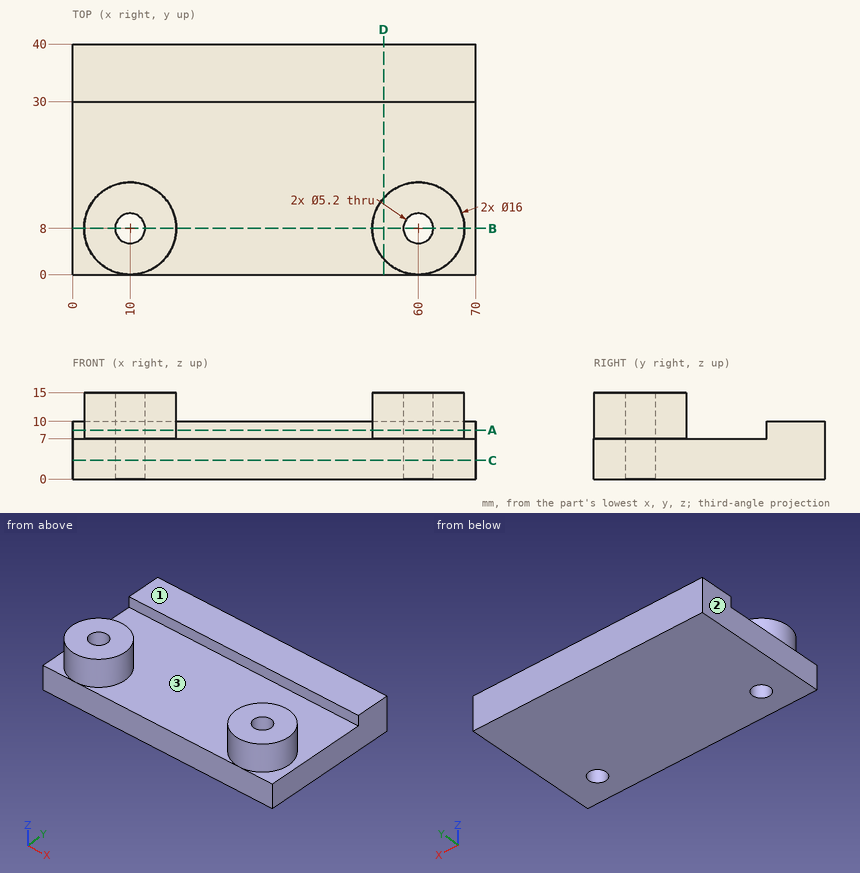
Could you check a few things on this drawing? It's one solid part, dimensions in mm from its lowest x, y, z. A direction names the side the tool comes from. Round coordinates to 2 decimals unless told otherwise and drop trailing zeros. Order: outer loops, then holes, each group sorted by start corner. A loop starts at its lowest first (then second) coordinate and runs counter-clockwise, first axis right, second up. Notation, with made-up numbers: M 4.5,-24.5 L 18.5,-24.5 A18 ccw 18.5,9.5 Z; hole C 74.25,54.25 d2. An arc over 180 degrees is marked long. Return JSON: item names as keys, results as strings. Group by question number.
1. I'm going to push flat-ended pins straight in: pin 1 Ø4 at (y, z) = (13.5, 11.5) entering from -X; pin 2 Ø9 at (x, y) = (26, 17.5) entering from +Z; pin 3 Ø8 at (x, y) = (48, 35.5) entering from +Z. Where does each tip first touch, or does it pass through?
2. If we section it at C-C on z = 3.25: List the corners of the cut face in (x, y) for me.
3. Please list where these lines run through material, in increasing order: probe 1 along Y at (x, z) = (10, 8.75); probe 2 along Y at (x, z) = (10, 6.5); probe 3 along Z at (x, y) = (49, 27).
4. If we section it at A-A on z = 8.5: List the corners of the cut face in (x, y) for me, then the cut area to 3 significant figures.
5. If we section it at B-B on y = 8: List the corners of the cut face in (x, z) for me.
6. If we section it at D-D on x = 54: List the corners of the cut face in (y, z) for me, then the cut area to 3 significant figures.
7. On a 3-axis mill with a long thin cutter (end or side, diameter ignored), from which of +Z, -Z, +X, -X, +Y, -Y can I reach the whole of each face in a straight line? I mean the marked faces 1, 2 and 3. Say none if no direction works.
Reply:
{
 "1": {"pin 1": "x = 2.81", "pin 2": "z = 7", "pin 3": "z = 10"},
 "2": {"outline": "M 0,0 L 70,0 L 70,40 L 0,40 Z; hole C 10,8 d5.2; hole C 60,8 d5.2"},
 "3": {"probe 1": "0 to 5.4, 10.6 to 16, 30 to 40", "probe 2": "0 to 5.4, 10.6 to 40", "probe 3": "0 to 7"},
 "4": {"outline": "M 0,30 L 70,30 L 70,40 L 0,40 Z; C 10,8 d16; C 60,8 d16; hole C 10,8 d5.2; hole C 60,8 d5.2", "area": "1,060 mm^2"},
 "5": {"outline": "M 0,0 L 7.4,0 L 7.4,15 L 2,15 L 2,7 L 0,7 Z; M 12.6,0 L 57.4,0 L 57.4,15 L 52,15 L 52,7 L 18,7 L 18,15 L 12.6,15 Z; M 62.6,0 L 70,0 L 70,7 L 68,7 L 68,15 L 62.6,15 Z"},
 "6": {"outline": "M 0,0 L 40,0 L 40,10 L 30,10 L 30,7 L 13.29,7 L 13.29,15 L 2.71,15 L 2.71,7 L 0,7 Z", "area": "395 mm^2"},
 "7": {"face 1": "+Z, +X, -X, +Y", "face 2": "+Z, -Z, -X, +Y, -Y", "face 3": "+Z"}
}
